Design review of the part built by this model. Coordinates are the model's own, in mm. Face numbers are marked on the shaded views. A direction names the side the tool comes from. Coordinates: 2 decimals unless noted, no trailing zeros. Write each loop counter-clockwise with the first axis right and the second up, starting at its lowest first coordinate (ties: lowest second). Pieces come first, ordered by that corner, then holes. Notation, with made-up numbers: (-4.75, 12.25) -> (13.25, 12.25) arc R11 cw to (13.25, 20.25) -> close; hole circle Ø8 at (3, 17.25). An arc over 180 degrees is marked (long way). Answer in a Markdown table with one row per item. Add a question column.
Item 1: Take a section at C-C, the plane x = 1.5. Write out the cut boundary in (y, z).
Item 2: Take a section at D-D, the plane z = 5. Write out the cut boundary in (x, y).
Item 3: Take a section at A-A, the plane y = 0. Give the number of separate pieces and of enclosed holes in the cut face, and give its area (3 significant figures).
Item 4: To check wall thickness, follow line 1 (Z direction, x = -16, y = 3.75); line 2 (Y direction, x = 0, z = 17); line 3 (Z direction, x = 10, y = -5). State the ranges of each line that lie inside material, in increasing order.
Item 5: Draft analysis for pull direction X (two halves, no side actions). For the marked faces 5, 6 and 7, state which applies: released by +X, released by -X, zero draft, split by the parting line, or undercut.
Item 6: Take a section at B-B, the plane x = -20. Write out the cut boundary in (y, z).
Item 7: Clearance check with flat-ended pins moving along their axes: P1, Ø6, axis at x = -14, y = 3, coming from the -Z side; P2, Ø1.9, axis at x = -1.5, z = -8.5, coming from the -Y side; P3, Ø3, axis at x = -14.5, y = 6.5, coming from the -Z side; P4, Ø2, axis at x = 3.5, y = 3, coming from the +Z side. State where each tip first meets the part, or that it passes through.
Item 8: For the marked faces 1, 2, 3 and 4, list the 3-axis set-ups (+Z, -Z, +X, -X, +Y, -Y) from which the entire face can be reached by the end or side of a thin tool; tool diameter is ignored.
Autodesk Inventor part; units mm, degrees
ref_plane "YZ Plane" through (0, 0, 0) normal (1, 0, 0) x (0, 1, 0)
ref_plane "XZ Plane" through (0, 0, 0) normal (0, 1, 0) x (-1, 0, 0)
ref_plane "XY Plane" through (0, 0, 0) normal (0, 0, 1) x (1, 0, 0)
sketch "Sketch12" plane through (0, 0, 0) normal (0, 0, 1) x (1, 0, 0)
  line L0 (-7.4168, 0) -> (7.4168, 0) construction
  line L1 (-7.4168, -9.0424) -> (7.4168, -9.0424)
  line L2 (7.4168, 9.0424) -> (-7.4168, 9.0424)
  arc A0 (-7.4168, 9.0424) -> (-7.4168, -9.0424) centre (-7.4168, 0) ccw
  arc A1 (7.4168, -9.0424) -> (7.4168, 9.0424) centre (7.4168, 0) ccw
  circle A2 centre (-20.0152, 0) radius 1.4605
  line L3 (0, 0) -> (0, -9.0424)
  circle A3 centre (-20.0152, 0) radius 3.4798
  line L4 (-21.5516, -3.1222) -> (-11.4093, -8.1133)
  line L5 (-21.5516, 3.1222) -> (-11.4093, 8.1133)
  circle A4 centre (20.0152, 0) radius 1.4605
  circle A5 centre (20.0152, 0) radius 3.4798
  line L6 (21.5516, -3.1222) -> (11.4093, -8.1133)
  line L7 (21.5516, 3.1222) -> (11.4093, 8.1133)
  point P0 (16.4592, 0)
  point P1 (-16.4592, 0)
  point P2 (11.4093, -8.1133)
  point P3 (11.4093, 8.1133)
  dimension "d107" = 32.9184
  dimension "d108" = 18.0848
  dimension "d109" = 40.0304
  dimension "d110" = 2.921
  dimension "d111" = 46.99
extrude "Extrusion1" add sketch "Sketch12" along normal mid plane 1.9558
sketch "Sketch13" plane through (0, 0, 0.9779) normal (0, 0, 1) x (1, 0, 0)
  arc A0 (-7.4168, 9.0424) -> (-7.4168, -9.0424) centre (-7.4168, 0) ccw
  arc A1 (7.4168, -9.0424) -> (7.4168, 9.0424) centre (7.4168, 0) ccw
  line L0 (7.4168, 9.0424) -> (-7.4168, 9.0424)
  line L1 (-7.4168, -9.0424) -> (7.4168, -9.0424)
  point P0 (0, 0)
extrude "Extrusion2" add sketch "Sketch13" along normal blind 10.414
sketch "Sketch14" plane through (0, 0, -0.9779) normal (0, 0, -1) x (-1, 0, 0)
  line L0 (7.4168, -9.0424) -> (-7.4168, -9.0424)
  arc A0 (-7.4168, 9.0424) -> (-7.4168, -9.0424) centre (-7.4168, 0) ccw
  line L1 (-7.4168, 9.0424) -> (7.4168, 9.0424)
  arc A1 (7.4168, -9.0424) -> (7.4168, 9.0424) centre (7.4168, 0) ccw
  point P0 (0, 0)
extrude "Extrusion3" add sketch "Sketch14" along normal blind 10.0965
sketch "Sketch15" plane through (0, 0, -11.0744) normal (0, 0, -1) x (-1, 0, 0)
  line L0 (-7.4168, -9.0424) -> (7.4168, -9.0424)
  arc A0 (7.4168, -9.0424) -> (7.4168, 9.0424) centre (7.4168, 0) ccw
  line L1 (7.4168, 9.0424) -> (-7.4168, 9.0424)
  arc A1 (-7.4168, 9.0424) -> (-7.4168, -9.0424) centre (-7.4168, 0) ccw
  line L2 (7.4168, -8.0137) -> (-7.4168, -8.0137)
  arc A2 (-7.4168, 8.0137) -> (-7.4168, -8.0137) centre (-7.4168, 0) ccw
  line L3 (-7.4168, 8.0137) -> (7.4168, 8.0137)
  arc A3 (7.4168, -8.0137) -> (7.4168, 8.0137) centre (7.4168, 0) ccw
  point P0 (0, 0)
  dimension "d118" = 16.0274
extrude "Extrusion4" cut sketch "Sketch15" against normal blind 3.8862
sketch "Sketch16" plane through (0, 0, -11.0744) normal (0, 0, -1) x (-1, 0, 0)
  arc A0 (7.4168, -8.0137) -> (7.4168, 8.0137) centre (7.4168, 0) ccw
  line L0 (7.4168, 8.0137) -> (-7.4168, 8.0137)
  arc A1 (-7.4168, 8.0137) -> (-7.4168, -8.0137) centre (-7.4168, 0) ccw
  line L1 (-7.4168, -8.0137) -> (7.4168, -8.0137)
  circle A2 centre (7.4168, 0) radius 4.7625
  circle A3 centre (-7.4168, 0) radius 4.7625
  point P0 (0, 0)
  dimension "d121" = 9.525
extrude "Extrusion5" add sketch "Sketch16" along normal blind 0.254 contours A2 | A3
sketch "Sketch17" plane through (0, 0, 11.3919) normal (0, 0, 1) x (1, 0, 0)
  line L0 (-7.4168, -9.0424) -> (7.4168, -9.0424)
  line L1 (2.54, -8.1534) -> (-2.54, -8.1534) construction
  line L2 (2.54, -7.5184) -> (-2.54, -7.5184)
  line L3 (-2.54, -8.7884) -> (2.54, -8.7884)
  arc A0 (2.54, -8.7884) -> (2.54, -7.5184) centre (2.54, -8.1534) ccw
  arc A1 (-2.54, -7.5184) -> (-2.54, -8.7884) centre (-2.54, -8.1534) ccw
  point P0 (0, 0)
  point P1 (0, -8.1534)
  point P2 (0, -8.7884)
  point P3 (0, -9.0424)
  dimension "d124" = 5.08
  dimension "d125" = 0.254
  dimension "d126" = 1.27
extrude "Extrusion6" add sketch "Sketch17" along normal blind 38.1
equation "\"BendRadius\" = Thickness"
equation "\"BendReliefWidth\" = Thickness"
equation "\"BendReliefDepth\" = 0.5 * Thickness"
equation "\"CornerReliefSize\" = 4 * Thickness"
equation "\"MinimumRemnant\" = 2 * Thickness"
equation "\"TransitionRadius\" = BendRadius"
equation "\"JacobiRadiusSize\" = BendRadius"
equation "\"GapSize\" = Thickness"
properties part number "Cage Sensor" material "Steel, Mild"
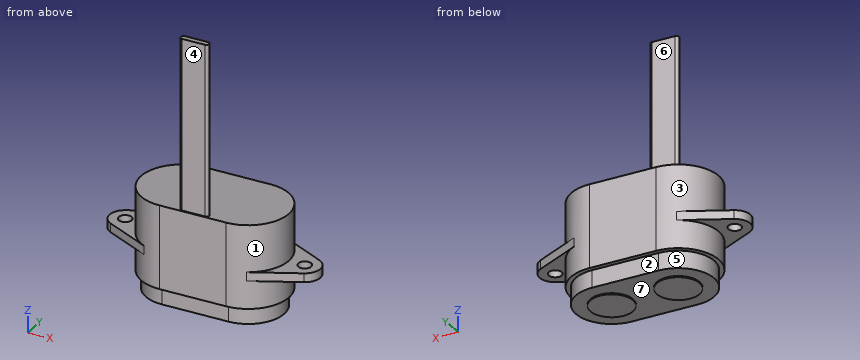
Answers:
| question | item | result |
|---|---|---|
| 1 | outline | (-9.04, -7.19) -> (-8.01, -7.19) -> (-8.01, -11.07) -> (8.01, -11.07) -> (8.01, -7.19) -> (9.04, -7.19) -> (9.04, 11.39) -> (-7.52, 11.39) -> (-7.52, 49.49) -> (-8.79, 49.49) -> (-8.79, 11.39) -> (-9.04, 11.39) -> close |
| 2 | outline | (-7.42, -9.04) -> (7.42, -9.04) arc R9.04 ccw to (7.42, 9.04) -> (-7.42, 9.04) arc R9.04 ccw to start |
| 3 | separate pieces | 3 |
| 3 | enclosed holes | 0 |
| 3 | area | 752 mm^2 |
| 4 | line 1 | z = -0.98 to 0.98 |
| 4 | line 2 | y = -8.79 to -7.52 |
| 4 | line 3 | z = -11.07 to 11.39 |
| 5 | face 5 | released by -X |
| 5 | face 6 | zero draft |
| 5 | face 7 | undercut |
| 6 | outline | (-3.89, -0.98) -> (-1.46, -0.98) -> (-1.46, 0.98) -> (-3.89, 0.98) -> close; (1.46, -0.98) -> (3.89, -0.98) -> (3.89, 0.98) -> (1.46, 0.98) -> close |
| 7 | P1 | stops at z = -11.33 |
| 7 | P2 | stops at y = -8.01 |
| 7 | P3 | stops at z = -7.19 |
| 7 | P4 | stops at z = 11.39 |
| 8 | face 1 | +X |
| 8 | face 2 | -Z, +X, -X, +Y |
| 8 | face 3 | -X |
| 8 | face 4 | +Z, +X, -X, -Y |
